Autodesk Inventor part; units mm, degrees
ref_plane "YZ Plane" through (0, 0, 0) normal (1, 0, 0) x (0, 1, 0)
ref_plane "XZ Plane" through (0, 0, 0) normal (0, 1, 0) x (-1, 0, 0)
ref_plane "XY Plane" through (0, 0, 0) normal (0, 0, 1) x (1, 0, 0)
sketch "Sketch1" plane through (0, 0, 0) normal (0, 1, 0) x (-1, 0, 0)
  circle A0 centre (0, 0) radius 25.4
  dimension "d0" = 50.8
extrude "Extrusion1" add sketch "Sketch1" along normal blind 6.35
sketch "Sketch2" plane through (0, 6.35, 0) normal (0, 1, 0) x (1, 0, 0)
  circle A0 centre (0, 0) radius 19.05
  dimension "d3" = 38.1
extrude "Extrusion2" add sketch "Sketch2" along normal blind 3.175
sketch "Sketch3" plane through (0, 9.525, 0) normal (0, 1, 0) x (1, 0, 0)
  circle A0 centre (0, 0) radius 25.4
  dimension "d6" = 50.8
extrude "Extrusion3" add sketch "Sketch3" along normal blind 6.35
sketch "Sketch5" plane through (0, 15.875, 0) normal (0, 1, 0) x (1, 0, 0)
  circle A0 centre (0, 0) radius 3
  dimension "d12" = 6
extrude "Extrusion5" cut sketch "Sketch5" against normal blind 3.175
properties part number "Drive_Wheel"
The listing builds one solid part. Answer for the finished solid, in the listing's coordinates (mm). A direction names the side the tool comes from. Round coordinates to 2 decimals unless told otherwise and drop trailing zeros. Loops run counter-clockwise (first coordinate to the right, second up) from the corner with the lowest first, then second, coordinate; pieces in that order, holes last. Notation, with made-up numbers: M 12,-36 L 43,-36 A30 ccw 43,-7 Z; hole C 69.25,46 d7. An arc over 180 degrees is marked long. Write each question's results on one line, items separated by ' | '. Start each with the question number.
1) Find section C-C on x = 0. Write down the section's boundary in (y, z) (3 decimals).
2) Find section B-B on z = -21.5. Write down the section's boundary in (x, y) (3 decimals).
3) Determine the mould class of faces 4 (the cylindrical face through (-5.506, 12.656, -24.796)), 5 (the flat face through (-4, 6.35, 19)), 6 (the flat face through (5, 15.875, 0)), 7 (the flat face through (0, 0, 0)) for opening direction Y: pulls with the +Y half, pulls with the -Y half, needs draft (parallel to the pull), parting line crosses it, or undercut.
4) Find section D-D on y = 14.25. Write down the section's boundary in (x, z).
5) Each of these flat-tipped pins is pushed along its axis until it touches: pin 1 (2 mm diameter, centred on y = 2, z = -12, fed in from +X); pin 2 (1.5 mm diameter, centred on x = 19.5, z = -5.5, fed in from -Y); pin 3 (5 mm diameter, centred on x = 0, z = 0, fed in from +Y); pin 4 (3 mm diameter, centred on y = 11, z = 19, fed in from +X). Where does it stop, or does it pass through?
6) Straight lines are drawn through the part: probe 1 along Y at (x, z) = (15.5, -17.5) (3 decimals); probe 2 along X at (y, z) = (13.75, 0). For each, find the intervals that lie inside material, in ascending order.
7) Find section A-A on x = 22. Write down the section's boundary in (y, z) (3 decimals), plus the area to 3 significant figures.
8) Which of the six approach directions +Z, -Z, +X, -X, +Y, -Y give full straight-line access (tool end or side, diameter ignored) to faces 1 (the flat face through (0, 12.7, 0)), 2 (the cylindrical face through (5.506, 3.131, 24.796)), 3 (the flat face through (4, 9.525, -19))?
Final values:
1) outline: M 0,-25.4 L 6.35,-25.4 L 6.35,-19.05 L 9.525,-19.05 L 9.525,-25.4 L 15.875,-25.4 L 15.875,-3 L 12.7,-3 L 12.7,3 L 15.875,3 L 15.875,25.4 L 9.525,25.4 L 9.525,19.05 L 6.35,19.05 L 6.35,25.4 L 0,25.4 Z
2) outline: M -13.524,0 L 13.524,0 L 13.524,6.35 L -13.524,6.35 Z; M -13.524,9.525 L 13.524,9.525 L 13.524,15.875 L -13.524,15.875 Z
3) face 4: needs draft | face 5: undercut | face 6: pulls with the +Y half | face 7: pulls with the -Y half
4) outline: C 0,0 d50.8; hole C 0,0 d6
5) pin 1: x = 22.89 | pin 2: y = 0 | pin 3: y = 12.7 | pin 4: x = 18.41
6) probe 1: 0 to 6.35, 9.525 to 15.875 | probe 2: -25.4 to -3, 3 to 25.4
7) outline: M 0,-12.695 L 6.35,-12.695 L 6.35,12.695 L 0,12.695 Z; M 9.525,-12.695 L 15.875,-12.695 L 15.875,12.695 L 9.525,12.695 Z | area: 322 mm²
8) face 1: +Y | face 2: +Y, -Y | face 3: none
